Autodesk Inventor part; units mm, degrees
ref_plane "Work Plane1" through (0, 0, 50) normal (0, 0, 1) x (1, 0, 0)
ref_plane "YZ Plane" through (0, 0, 0) normal (1, 0, 0) x (0, 1, 0)
ref_plane "XZ Plane" through (0, 0, 0) normal (0, 1, 0) x (-1, 0, 0)
sketch "Sketch2" plane through (0, 0, 0) normal (0, 1, 0) x (-1, 0, 0)
  line L0 (-50, 0) -> (-50, 5)
  line L1 (50, 5) -> (50, 0)
  arc A0 (38.5, 0) -> (-38.5, 0) centre (0, 0) ccw
  line L2 (50, 5) -> (35.3035, 25.4148)
  line L3 (-50, 5) -> (-35.3035, 25.4148)
  line L4 (50, 0) -> (38.5, 0)
  line L5 (-38.5, 0) -> (-50, 0)
  line L6 (43.2117, 5) -> (50, 5)
  arc A1 (35.3035, 25.4148) -> (-35.3035, 25.4148) centre (0, 0) ccw
  point P0 (50, 2.5)
  dimension "d0" = 77
  dimension "d2" = 5
  dimension "d3" = 100
  dimension "d4" = 50
extrude "Extrusion1" add sketch "Sketch2" along normal blind 14
ref_plane "Work Plane1" through (0, 0, 50) normal (0, 0, 1) x (1, 0, 0)
sketch "Sketch3" plane through (0, 0, 50) normal (0, 0, 1) x (1, 0, 0)
  line L0 (-38.5, 0) -> (-38.5, 14)
  circle A0 centre (44, 7) radius 2.5
  circle A1 centre (44, 7) radius 3.5
  line L1 (0, 0) -> (0, 17.8681)
  circle A2 centre (-44, 7) radius 2.5
  circle A3 centre (-44, 7) radius 3.5
  line L2 (35.3035, 14) -> (50, 14)
  dimension "d10" = 1
  dimension "d11" = 44
  dimension "d12" = 7
extrude "Extrusion2" cut sketch "Sketch3" against normal blind 45
extrude "Extrusion3" cut sketch "Sketch3" against normal blind 60 contours A0 | A2
properties part number "clamp" material "Polyethylene, High Density"
Can you work these out from the model? Positions are in its coordinate system, mm. A direction names the side the tool comes from. Coordinates: 2 decimals unless noted, no trailing zeros. Write each loop counter-clockwise with the first axis right and the second up, starting at its lowest first coordinate (ties: lowest second). Pieces come first, ordered by that corner, then holes. Notation, with made-up numbers: (17, 51) - (55, 51) arc R16 ccw to (55, 62) - close; hole circle Ø11 at (-38, 64). An arc over 180 degrees is marked (long way). Return JSON: item names as keys, results as strings. Group by question number.
Item 1: I'm going to push flat-ended pins straight in: pin 1 Ø1.5 at (y, z) = (5.5, 19.5) entering from +X; pin 2 Ø8 at (x, y) = (44, 7) entering from +Z; pin 3 Ø5 at (x, y) = (32.5, 11.5) entering from +Z. Where does each tip first touch, or does it pass through?
Item 2: We'd pull the mould along X, two halves only. Please class faces 1 (the face through (0.577, 6.902, 43.496)), 2 (the face through (-41.69, 6.04, 2.53)), 3 (the face through (50, 7, 2)): pulls with the +X half, pulls with the -X half, needs draft (parallel to the pull), parting line crosses it, or undercut.
Item 3: Please list where these lines run through material, in increasing order: probe 1 along Y at (x, z) = (44, 3); probe 2 along Y at (x, z) = (-44, 11.5); probe 3 along X at (y, z) = (0.75, 29).
Item 4: If we section it at B-B (z = 12.5): Write out the boundary of the cut face in (x, y).
Item 5: If we section it at D-D (x = -13): Write out the boundary of the cut face in (y, z), then the cut area to 3 significant figures.
Item 6: If we section it at A-A (x = 44): Write out the boundary of the cut face in (y, z).
Item 7: Which directions (+Z, -Z, +X, -X, +Y, -Y) give clear straight access to the entire face, cutting with the end or side of a thin tool? Please do faces 4 (the face through (-42, 5, 5)), 5 (the face through (8, 0, 38)).
Item 8: If we section it at C-C (x = 0): Write out the boundary of the cut face in (y, z), then the cut area to 3 significant figures.
Return value:
{
 "1": {"pin 1": "stops at x = 40.1", "pin 2": "stops at z = 18.89", "pin 3": "stops at z = 31.5"},
 "2": {"face 1": "parting line crosses it", "face 2": "undercut", "face 3": "pulls with the +X half"},
 "3": {"probe 1": "y = 0 to 4.5, 9.5 to 14", "probe 2": "y = 0 to 3.5, 10.5 to 14", "probe 3": "x = -32.42 to -25.32, 25.32 to 32.42"},
 "4": {"outline": "(-44.6, 0) - (-36.41, 0) - (-36.41, 14) - (-44.6, 14) - (-44.6, 10.45) arc R3.5 cw (long way) to (-44.6, 3.55) - close; (36.41, 0) - (44.6, 0) - (44.6, 3.55) arc R3.5 cw (long way) to (44.6, 10.45) - (44.6, 14) - (36.41, 14) - close"},
 "5": {"outline": "(0, 36.24) - (14, 36.24) - (14, 41.51) - (0, 41.51) - close", "area": "73.8 mm^2"},
 "6": {"outline": "(0, 0) - (4.5, 0) - (4.5, 5) - (3.5, 5) - (3.5, 13.33) - (0, 13.33) - close; (9.5, 0) - (14, 0) - (14, 13.33) - (10.5, 13.33) - (10.5, 5) - (9.5, 5) - close"},
 "7": {"face 4": "+Z", "face 5": "+Z, -Z, +X, -X, -Y"},
 "8": {"outline": "(0, 38.5) - (14, 38.5) - (14, 43.5) - (0, 43.5) - close", "area": "70.0 mm^2"}
}
